from build123d import *

# Parameters (mm, degrees)
SKETCH2_W                        = 30
SKETCH2_H                        = 18
EXTRUDE_BASE_DEPTH               = 3
SKETCH3_R                        = 9
EXTRUDE_CYLINDER_DEPTH           = 5
SKETCH4_W                        = 40
SKETCH4_H                        = 18
EXTRUDE_PHONE_FLOOR_DEPTH        = 4
SKETCH5_W                        = 40
SKETCH5_H                        = 6
EXTRUDE_PHONE_ROOF_DEPTH         = 18
CUT_PHONE_CRADLE_DEPTH           = 54.141321022
CUT_PHONE_CRADLE_DEPTH_BACK      = 54.141321022
CUT_RUBBER_BAND_HOLDERS_REACH    = 51.487
SKETCH7_W                        = 3
SKETCH7_H                        = 3
FILLET_RUBBER_BAND_HOLDERS_R     = 1.5
FILLET_RUBBER_BAND_HOLDERS_R_2   = 0.5
SKETCH8_W                        = 30
SKETCH8_H                        = 62
EXTRUDE_BASE_EXTENSION_DEPTH     = 3
EXTRUDE_CYLINDER_EXTENSION_DEPTH = 5
SKETCH10_W                       = 30
SKETCH10_H                       = 62
EXTRUDE_FLOOR_EXTENSION_DEPTH    = 2
FILLET1_R                        = 10


# Some blends are built 0.0001 mm under size
with BuildPart() as part:
    # Sketch2 → Extrude-Base (new body)
    with BuildSketch(Plane(origin=(0, 0, 0), x_dir=(1, 0, 0), z_dir=(0, 1, 0))):
        with Locations((15, -9)):
            Rectangle(SKETCH2_W, SKETCH2_H)
    extrude(amount=EXTRUDE_BASE_DEPTH)

    # Sketch3 → Extrude-Cylinder (add)
    with BuildSketch(Plane(origin=(0, 3, 0), x_dir=(1, 0, 0), z_dir=(0, 1, 0))):
        with Locations(Location((15, -9, 0), (0, 0, 270))):
            Circle(SKETCH3_R)
    extrude(amount=EXTRUDE_CYLINDER_DEPTH)

    # Sketch4 → Extrude-Phone Floor (add)
    with BuildSketch(Plane(origin=(0, 8, 0), x_dir=(1, 0, 0), z_dir=(0, 1, 0))):
        with Locations((15, -9)):
            Rectangle(SKETCH4_W, SKETCH4_H)
    extrude(amount=EXTRUDE_PHONE_FLOOR_DEPTH)

    # Sketch5 → Extrude-Phone Roof (add)
    with BuildSketch(Plane(origin=(0, 12, 0), x_dir=(1, 0, 0), z_dir=(0, 1, 0))):
        with Locations((15, -15)):
            Rectangle(SKETCH5_W, SKETCH5_H)
    extrude(amount=EXTRUDE_PHONE_ROOF_DEPTH)

    # Sketch6 → Cut-Phone Cradle (cut, two sides: drawn at the far end of the back side and taken through both)
    with BuildSketch(Plane(origin=(35, 0, 0), x_dir=(0, 0, -1), z_dir=(1, 0, 0)).offset(-CUT_PHONE_CRADLE_DEPTH_BACK)):
        with BuildLine():
            Line((-12, 12), (-12, 28))
            ThreePointArc((-12, 28), (-15, 20), (-12, 12))
        make_face()
    extrude(amount=CUT_PHONE_CRADLE_DEPTH + CUT_PHONE_CRADLE_DEPTH_BACK, mode=Mode.SUBTRACT)

    # Sketch7 → Cut-Rubber Band Holders (cut, up to next)
    with BuildSketch(Plane.XZ, mode=Mode.PRIVATE) as cut_rubber_band_holders_sk1:
        with Locations((24.5, 16.5)):
            Rectangle(SKETCH7_W, SKETCH7_H)
    cut_rubber_band_holders_tool1 = extrude(cut_rubber_band_holders_sk1.sketch, amount=-CUT_RUBBER_BAND_HOLDERS_REACH, mode=Mode.PRIVATE) & part.part
    # Sketch7 → Cut-Rubber Band Holders (cut, up to next)
    with BuildSketch(Plane.XZ, mode=Mode.PRIVATE) as cut_rubber_band_holders_sk2:
        with Locations((5.5, 16.5)):
            Rectangle(SKETCH7_W, SKETCH7_H)
    cut_rubber_band_holders_tool2 = extrude(cut_rubber_band_holders_sk2.sketch, amount=-CUT_RUBBER_BAND_HOLDERS_REACH, mode=Mode.PRIVATE) & part.part
    add(cut_rubber_band_holders_tool1.solids().sort_by_distance((24.5, 0, 16.5))[0], mode=Mode.SUBTRACT)
    add(cut_rubber_band_holders_tool2.solids().sort_by_distance((5.5, 0, 16.5))[0], mode=Mode.SUBTRACT)

    # Fillet-Rubber Band Holders
    fillet_rubber_band_holders_edges = [part.edges().sort_by_distance(p)[0] for p in [
        (26, 1.5, 15),
        (7, 1.5, 15),
        (23, 1.5, 15),
        (4, 1.5, 15),
    ]]
    fillet(fillet_rubber_band_holders_edges, radius=FILLET_RUBBER_BAND_HOLDERS_R - 0.0001)  # a hair under: the kernel refuses the full size
    fillet_rubber_band_holders_2_edges = [part.edges().sort_by_distance(p)[0] for p in [
        (24.5, 3, 15),
        (24.5, 0, 15),
        (5.5, 0, 15),
        (5.5, 3, 15),
        (6.560689461, 3, 15.439310539),
        (4.439310539, 3, 15.439310539),
        (4.439310539, 0, 15.439310539),
        (6.560689461, 0, 15.439310539),
        (23.439310539, 0, 15.439310539),
        (25.560689461, 0, 15.439310539),
        (25.560689461, 3, 15.439310539),
        (23.439310539, 3, 15.439310539),
    ]]
    fillet(fillet_rubber_band_holders_2_edges, radius=FILLET_RUBBER_BAND_HOLDERS_R_2)

    # Sketch8 → Extrude-Base Extension (add)
    with BuildSketch(Plane.XZ):
        with Locations((15, -31)):
            Rectangle(SKETCH8_W, SKETCH8_H)
    extrude(amount=-EXTRUDE_BASE_EXTENSION_DEPTH)

    # Sketch9 → Extrude-Cylinder Extension (add)
    with BuildSketch(Plane(origin=(0, 3, 0), x_dir=(1, 0, 0), z_dir=(0, 1, 0))):
        with BuildLine():
            Line((24, -9), (24, 53))
            ThreePointArc((24, 53), (15, 62), (6, 53))
            Line((6, 53), (6, -9))
            ThreePointArc((6, -9), (15, 0), (24, -9))
        make_face()
    extrude(amount=EXTRUDE_CYLINDER_EXTENSION_DEPTH)

    # Sketch10 → Extrude-Floor Extension (add)
    with BuildSketch(Plane(origin=(0, 8, 0), x_dir=(1, 0, 0), z_dir=(0, 1, 0))):
        with Locations((15, 31)):
            Rectangle(SKETCH10_W, SKETCH10_H)
    extrude(amount=EXTRUDE_FLOOR_EXTENSION_DEPTH)

    # Fillet1
    # the kernel refuses this fillet: 10 mm, written as the material it adds along each edge
    with BuildSketch(Plane(origin=(0, 8, 0), x_dir=(0, 0, -1), z_dir=(0, 1, 0))) as fillet1_piece_1:
        with BuildLine():
            CenterArc((8.660254038, 10), FILLET1_R, 210, 60)
            Line((0, 5), (-0.173205081, 4.9))
            ThreePointArc((-0.173205081, 4.9), (-0.2, 2.5), (-0.2, 0))
            Line((-0.2, 0), (0, -0.2))
            Line((0, -0.2), (8.660254038, -0.2))
            Line((8.660254038, -0.2), (8.660254038, 0))
        make_face()
    extrude(amount=2)
    with BuildSketch(Plane(origin=(0, 10, 0), x_dir=(0, 0, -1), z_dir=(1, 0, 0))) as fillet1_piece_2:
        with BuildLine():
            CenterArc((6, 10), FILLET1_R, 233.130102354, 36.869897646)
            Line((0, 2), (-0.12, 1.84))
            ThreePointArc((-0.12, 1.84), (-0.2, 1), (-0.2, 0))
            Line((-0.2, 0), (0, -0.2))
            Line((0, -0.2), (6, -0.2))
            Line((6, -0.2), (6, 0))
        make_face()
    extrude(amount=30)
    with BuildSketch(Plane(origin=(30, 8, 0), x_dir=(0, 0, -1), z_dir=(0, 1, 0))) as fillet1_piece_3:
        with BuildLine():
            CenterArc((8.660254038, -10), FILLET1_R, 90, 60)
            Line((0, -5), (-0.173205081, -4.9))
            ThreePointArc((-0.173205081, -4.9), (-0.2, -2.5), (-0.2, 0))
            Line((-0.2, 0), (0, 0.2))
            Line((0, 0.2), (8.660254038, 0.2))
            Line((8.660254038, 0.2), (8.660254038, 0))
        make_face()
    extrude(amount=2)
    with BuildSketch(Plane(origin=(-15, 10, 0), x_dir=(0, 0, -1), z_dir=(1, 0, 0))) as fillet1_piece_4a_section:
        with BuildLine():
            CenterArc((6, 10), FILLET1_R, 233.130102354, 36.869897646)
            Line((0, 2), (-0.12, 1.84))
            ThreePointArc((-0.12, 1.84), (-0.2, 1), (-0.2, 0))
            Line((-0.2, 0), (0, -0.2))
            Line((0, -0.2), (6, -0.2))
            Line((6, -0.2), (6, 0))
        make_face()
    fillet1_piece_4a = extrude(amount=45, mode=Mode.PRIVATE)
    fillet1_piece_4a = split(fillet1_piece_4a, bisect_by=Plane(origin=(0, 10.452376795, -1.699345627), z_dir=(-1, 0, 0)), keep=Keep.TOP, mode=Mode.PRIVATE)
    fillet1_piece_4a = split(fillet1_piece_4a, bisect_by=Plane(origin=(-5, 10.452376795, -1.699345627), z_dir=(1, 0, 0)), keep=Keep.TOP, mode=Mode.PRIVATE)
    with BuildSketch(Plane(origin=(0, 8, 0), x_dir=(0, 0, -1), z_dir=(0, 1, 0))) as fillet1_piece_4b_section:
        with BuildLine():
            CenterArc((8.660254038, 10), FILLET1_R, 210, 60)
            Line((0, 5), (-0.173205081, 4.9))
            ThreePointArc((-0.173205081, 4.9), (-0.2, 2.5), (-0.2, 0))
            Line((-0.2, 0), (0, -0.2))
            Line((0, -0.2), (8.660254038, -0.2))
            Line((8.660254038, -0.2), (8.660254038, 0))
        make_face()
    fillet1_piece_4b = extrude(amount=23.650635095, mode=Mode.PRIVATE)
    fillet1_piece_4b = split(fillet1_piece_4b, bisect_by=Plane(origin=(-1.295167111, 10, -2.163104458), z_dir=(0, 1, 0)), keep=Keep.TOP, mode=Mode.PRIVATE)
    fillet1_piece_4b = split(fillet1_piece_4b, bisect_by=Plane(origin=(-1.295167111, 12, -2.163104458), z_dir=(0, -1, 0)), keep=Keep.TOP, mode=Mode.PRIVATE)
    fillet1_piece_4 = fillet1_piece_4a & fillet1_piece_4b
    add(fillet1_piece_4)
    with BuildSketch(Plane(origin=(0, 10, 0), x_dir=(0, 0, -1), z_dir=(1, 0, 0))) as fillet1_piece_5a_section:
        with BuildLine():
            CenterArc((6, 10), FILLET1_R, 233.130102354, 36.869897646)
            Line((0, 2), (-0.12, 1.84))
            ThreePointArc((-0.12, 1.84), (-0.2, 1), (-0.2, 0))
            Line((-0.2, 0), (0, -0.2))
            Line((0, -0.2), (6, -0.2))
            Line((6, -0.2), (6, 0))
        make_face()
    fillet1_piece_5a = extrude(amount=45, mode=Mode.PRIVATE)
    fillet1_piece_5a = split(fillet1_piece_5a, bisect_by=Plane(origin=(30, 10.452376795, -1.699345627), z_dir=(1, 0, 0)), keep=Keep.TOP, mode=Mode.PRIVATE)
    fillet1_piece_5a = split(fillet1_piece_5a, bisect_by=Plane(origin=(35, 10.452376795, -1.699345627), z_dir=(-1, 0, 0)), keep=Keep.TOP, mode=Mode.PRIVATE)
    with BuildSketch(Plane(origin=(30, 8, 0), x_dir=(0, 0, -1), z_dir=(0, 1, 0))) as fillet1_piece_5b_section:
        with BuildLine():
            CenterArc((8.660254038, -10), FILLET1_R, 90, 60)
            Line((0, -5), (-0.173205081, -4.9))
            ThreePointArc((-0.173205081, -4.9), (-0.2, -2.5), (-0.2, 0))
            Line((-0.2, 0), (0, 0.2))
            Line((0, 0.2), (8.660254038, 0.2))
            Line((8.660254038, 0.2), (8.660254038, 0))
        make_face()
    fillet1_piece_5b = extrude(amount=23.650635095, mode=Mode.PRIVATE)
    fillet1_piece_5b = split(fillet1_piece_5b, bisect_by=Plane(origin=(31.295167111, 10, -2.163104458), z_dir=(0, 1, 0)), keep=Keep.TOP, mode=Mode.PRIVATE)
    fillet1_piece_5b = split(fillet1_piece_5b, bisect_by=Plane(origin=(31.295167111, 12, -2.163104458), z_dir=(0, -1, 0)), keep=Keep.TOP, mode=Mode.PRIVATE)
    fillet1_piece_5 = fillet1_piece_5a & fillet1_piece_5b
    add(fillet1_piece_5)


solid = part.part
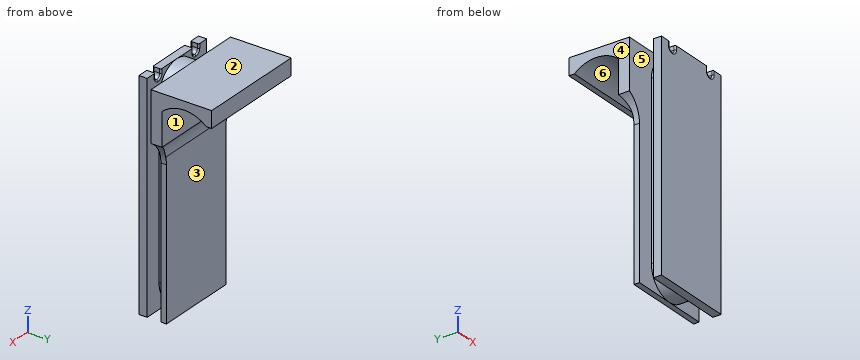
Can you work these out from the model? Positions are in its coordinate system, mm. Face numbers are marked on the shaded views. A direction names the side the tool comes from. Coordinates: 2 decimals unless noted, no trailing zeros. Write each loop counter-clockwise with the first axis right and the second up, starting at its lowest first coordinate (ties: lowest second). Pieces come first, ordered by that corner, then holes. Notation, with made-up numbers: (28.5, -13) -> (52.5, -13) arc R30 ccw to (52.5, 25) -> close; hole circle Ø8 at (83, 44.25). An arc over 180 degrees is marked (long way). Answer as CSV lines item,"result".
1) If we section it at C-C on y = 7: Please give me the cut outline in (x, z).
Check result:
outline,"(6, -53) arc R9 ccw to (24, -53) -> (24, 9) arc R9 ccw to (6, 9) -> close"
2) On a 3-axis mill with a long thin cutter (end or side, diameter ignored), from which of +Z, -Z, +X, -X, +Y, -Y can I reach the whole of each face in a straight line? I mean the marked faces 1 and 2. Say none if no direction works.
Check result:
face 1,"-Z, +X, -X, +Y"
face 2,"+Z, +X, -X, +Y, -Y"
3) If we section it at B-B on x = -2: Please give me the cut outline in (y, z), then the cut area to 3 significant figures.
Check result:
outline,"(8, -2.66) -> (10.57, -2.66) arc R10 cw to (12, 0) -> (12, 12) arc R12.17 cw to (28, 12) -> (30, 12) -> (30, 18) -> (8, 18) -> close"
area,"156 mm²"
4) If we section it at D-D on x = 12.5: Please give me the cut outline in (y, z), then the cut area to 3 significant figures.
Check result:
outline,"(0, -62) -> (3, -62) -> (3, -61.65) -> (8, -61.65) -> (8, -62) -> (10, -62) -> (10, -6) arc R10 cw to (12, 0) -> (12, 12) arc R12.17 cw to (28, 12) -> (30, 12) -> (30, 18) -> (8, 18) -> (8, 17.65) -> (3, 17.65) -> (3, 18) -> (0, 18) -> close"
area,"911 mm²"
5) If we mould it in two halves opening along Y, with no side actions, what happens to the marked faces 3, 4, 5 and 6? For each: +Y half, -Y half, draft (parallel to the pull), parting line (faces both ways), or undercut.
Check result:
face 3,"+Y half"
face 4,"draft"
face 5,"undercut"
face 6,"undercut"
6) If we section it at A-A on z = -50: Please give me the cut outline in (x, y), then the cut area to 3 significant figures.
Check result:
outline,"(0, 0) -> (30, 0) -> (30, 3) -> (24, 3) -> (24, 8) -> (30, 8) -> (30, 10) -> (0, 10) -> (0, 8) -> (6, 8) -> (6, 3) -> (0, 3) -> close"
area,"240 mm²"
7) If I drill on line 1 (Y direction, x = 24.5, z = -10); line 2 (Y direction, x = 5, z = 0.5); line 3 (Z direction, x = 13, y = 23.5), over which ranges is the centre line in solid material (lowest first)? Write a range as from..to.
Check result:
line 1,"0..3, 8..10"
line 2,"0..3, 8..12"
line 3,"14.49..18"
8) Will these pins go through, and if not, where does the flat tip stop? P1, Ø10, axis at x = 26.5, z = -15.5, coming from the -Y side; P2, Ø0.8, axis at y = 1.5, z = 17.5, coming from the +X side; P3, Ø1.5, axis at x = 0, z = -7, coming from the +Y side; P4, Ø2, axis at x = 29.5, y = 25.5, coming from the -Z side.
Check result:
P1,"y = 0"
P2,"x = 30"
P3,"y = 10"
P4,"z = 13.12"
